```python
from build123d import *

# Parameters (mm, degrees)
F1_DEPTH       = 37
F2_W           = 12
F2_H           = 2
F3_DEPTH       = 2
F4_W           = 16
F4_H           = 34
F5_DEPTH       = 3
F7_W           = 1
F7_H           = 10
F7_W_2         = 16
F7_H_2         = 2
F8_DEPTH       = 1.5
F9_SIZE        = 1
F10_R          = 1
F11_DEPTH      = 1.5
F11_DEPTH_BACK = 3


with BuildPart() as f1:
    # F0 (on Front) → F1 (new body)
    with BuildSketch(Plane.XZ):
        Polygon((-9, 1), (-8, 0), (8, 0), (9, 1), (9, 4), (6, 4), (6, 2), (-6, 2), (-6, 4), (-9, 4), align=None)
    extrude(amount=F1_DEPTH)

    # F2 (on face) → F3 (join)
    with BuildSketch(Plane(origin=(0, 0, 0), x_dir=(-1, 0, 0), z_dir=(0, 1, 0))):
        with Locations((0, 3)):
            Rectangle(F2_W, F2_H)
    extrude(amount=-F3_DEPTH)

    # F4 (on face) → F5 (cut)
    with BuildSketch(Plane.XY.offset(4)):
        with Locations((0, -18.5)):
            Rectangle(F4_W, F4_H)
    extrude(amount=-F5_DEPTH, mode=Mode.SUBTRACT)

    # F7 (on offset) → F8 (join, through all)
    with BuildSketch(Plane.XY.offset(2.5)):
        with Locations((-7.5, -6.5)):
            Rectangle(F7_W, F7_H)
        with Locations((7.5, -6.5)):
            Rectangle(F7_W, F7_H)
        with Locations((0, -22.5)):
            Rectangle(F7_W_2, F7_H_2)
    extrude(amount=-F8_DEPTH)

    # F9
    f9_edges = [f1.edges().sort_by_distance(p)[0] for p in [
        (0, 0, 0),
        (0, -37, 0),
    ]]
    chamfer(f9_edges, length=F9_SIZE)

    # F10 (on face) → F11 (join, two sides)
    with BuildSketch(Plane.XY.offset(4)) as f11_sk:
        with Locations((7.5, -35)):
            Circle(F10_R)
        with Locations((-7.5, -35)):
            Circle(F10_R)
        with Locations((-7.5, -1.5)):
            Circle(F10_R)
        with Locations((7.5, -1.5)):
            Circle(F10_R)
    extrude(amount=F11_DEPTH)
    extrude(f11_sk.sketch, amount=-F11_DEPTH_BACK)


solid = f1.part
```
Work out the finished part from the listing and answer in its coordinate system (mm). A direction names the side the tool comes from. Coordinates: 2 decimals unless noted, no trailing zeros. Order: outer loops, then holes, each group sorted by start corner. A loop starts at its lowest first (then second) coordinate and runs counter-clockwise, first axis right, second up. Notation, with made-up numbers: (-30, 76.25) - (15, 76.25) arc R36 cw to (15, 113.25) - close; hole circle Ø10 at (-2, 38.5). An arc over 180 degrees is marked (long way). Answer as a JSON object with one key per item and string values.
1. The mould has two halves that part along X. Classify faces 4 (the face through (9, -18, 2)), 5 (the face through (0, -1.5, 3)), 6 (the face through (-8, -1, 5.5)): +X half, -X half, draft (parallel to the pull), parting line (faces both ways), or undercut.
Output values:
{"face 4": "+X half", "face 5": "undercut", "face 6": "draft"}
2. Each of these flat-tipped pins is pushed along its axis until it touches: P1, Ø4, axis at x = -4.5, y = -10, coming from the +Z side; P2, Ø0.5, axis at x = -7.5, y = -8, coming from the +Z side. Where does it stop, or does it pass through?
Output values:
{"P1": "stops at z = 1", "P2": "stops at z = 2.5"}
3. Find section B-B on y = -26. Determine the outline of the cut face in (x, z).
Output values:
{"outline": "(-9, 1) - (-8, 0) - (8, 0) - (9, 1) - (9, 4) - (8, 4) - (8, 1) - (-8, 1) - (-8, 4) - (-9, 4) - close"}
4. Find section A-A on z = 1.5. Determine the outline of the cut face in (x, y).
Output values:
{"outline": "(-9, -37) - (9, -37) - (9, 0) - (-9, 0) - close; hole (-8, -34.13) arc R1 cw to (-6.63, -35.5) - (6.63, -35.5) arc R1 cw to (8, -34.13) - (8, -23.5) - (-8, -23.5) - close; hole (-8, -21.5) - (8, -21.5) - (8, -11.5) - (7, -11.5) - (7, -2.37) arc R1 cw to (6.5, -1.5) - (-6.5, -1.5) arc R1 cw to (-7, -2.37) - (-7, -11.5) - (-8, -11.5) - close"}
5. Find section D-D on z = 4.9. Determine the outline of the cut face in (x, y), plus the area to 3 significant figures.
Output values:
{"outline": "circle Ø2 at (-7.5, -35); circle Ø2 at (-7.5, -1.5); circle Ø2 at (7.5, -35); circle Ø2 at (7.5, -1.5)", "area": "12.6 mm²"}
6. Consider line 1 (Y direction, x = 3.75, z = 1.05); line 2 (X direction, y = -8, z = 1.2); line 3 (Y direction, x = 6.75, z = 2.05). Determine where each line is inside the solid, lowest interval first.
Output values:
{"line 1": "y = -37 to -35.5, -23.5 to -21.5, -1.5 to 0", "line 2": "x = -9 to -7, 7 to 9", "line 3": "y = -37 to -34.34, -23.5 to -21.5, -2.16 to 0"}
7. Find section C-C on x = -2.25. Determine the outline of the cut face in (y, z), plus the area to 3 significant figures.
Output values:
{"outline": "(-37, 1) - (-36, 0) - (-1, 0) - (0, 1) - (0, 4) - (-1.5, 4) - (-1.5, 1) - (-21.5, 1) - (-21.5, 2.5) - (-23.5, 2.5) - (-23.5, 1) - (-35.5, 1) - (-35.5, 2) - (-37, 2) - close", "area": "45.0 mm²"}
8. A tool of negligible diameter and unlimited length cuts with its end or side. For faces 1 (the face through (0, -18, 0)), 2 (the face through (0, -36, 2)), 3 (the face through (8.7, -15.7, 4)), from which of +Z, -Z, +X, -X, +Y, -Y can it reach the whole face along a straight path? Write none if from no direction.
Output values:
{"face 1": "-Z, +X, -X, +Y, -Y", "face 2": "+Z, -Y", "face 3": "+Z"}
